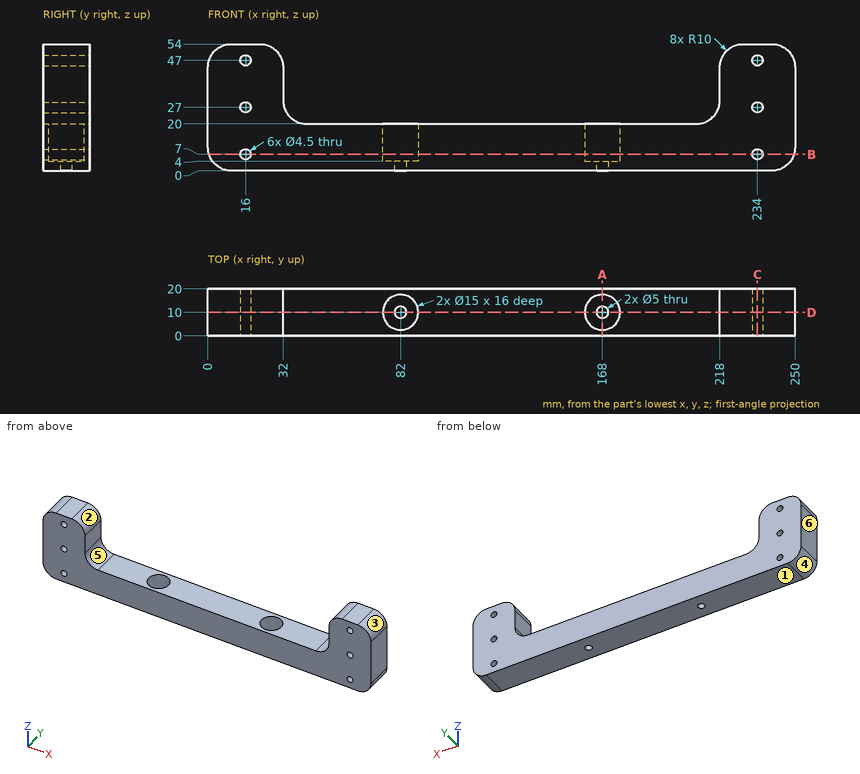
Can you work these out from the drawing? Everything is in mm from the part's minimum corner. A direction names the side the tool comes from. Give positions to 0.01 mm unless a question says otherwise; leave off trailing zeros. Order: outer loops, then holes, each group sorted by start corner. A loop starts at its lowest first (then second) coordinate and runs counter-clockwise, first axis right, second up. Notation, with made-up numbers: M -37,51 L -23,51 A30 cw -23,90 Z; hole C 65.25,-5.75 d7. An arc over 180 degrees is marked long. Use a Markdown table: item, result. Add a question column.
1. For pin 1 Ø5 at (y, z) = (17, 5.5) entering from +X; pin 2 Ø7.5 at (x, y) = (166.5, 9.5) entering from +Z, each with a flat end and sliding along its axis, tell me the tip position at first contact or that it passes through.
2. I need wall thicknesses on probe 1 along Z at (x, y) = (234, 15.25); probe 2 along X at (y, z) = (5.25, 33); probe 3 along Y at (x, z) = (168, 12). Which ranges of each line are inside material? Lowest first, please. Write a range as from..to.
3. Suppose I cut it at D-D (y = 10). Give the number of separate pieces and of enclosed holes in the cut face, and give its area (3 significant figures).
4. Suppose I cut it at A-A (x = 168). List the corners of the cut face in (y, z) for me, and give its area (3 significant figures).
5. Suppose I cut it at B-B (z = 7). List the corners of the cut face in (x, y) for me, and give its area (3 significant figures).
6. If we mould it in two halves opening along X, with no side actions, what happens to the marked faces 1, 2, 3 and 4? For each: +X half, -X half, draft (parallel to the pull), parting line (faces both ways), or undercut.
7. Suppose I cut it at C-C (x = 234). List the corners of the cut face in (y, z) for me, and give its area (3 significant figures).
8. On a 3-axis mill with a long thin cutter (end or side, diameter ignored), from which of +Z, -Z, +X, -X, +Y, -Y can I reach the whole of each face in a straight line? I mean the marked faces 5 and 6. Say none if no direction works.
Results list:
| question | item | result |
|---|---|---|
| 1 | pin 1 | stops at x = 249.8 |
| 1 | pin 2 | stops at z = 4 |
| 2 | probe 1 | z = 0..4.75, 9.25..24.75, 29.25..44.75, 49.25..54 |
| 2 | probe 2 | x = 0..32, 218..250 |
| 2 | probe 3 | y = 0..2.5, 17.5..20 |
| 3 | separate pieces | 3 |
| 3 | enclosed holes | 6 |
| 3 | area | 6,470 mm² |
| 4 | outline | M 0,0 L 7.5,0 L 7.5,4 L 2.5,4 L 2.5,20 L 0,20 Z; M 12.5,0 L 20,0 L 20,20 L 17.5,20 L 17.5,4 L 12.5,4 Z |
| 4 | area | 140 mm² |
| 5 | outline | M 0.46,0 L 13.75,0 L 13.75,20 L 0.46,20 Z; M 18.25,0 L 231.75,0 L 231.75,20 L 18.25,20 Z; M 236.25,0 L 249.54,0 L 249.54,20 L 236.25,20 Z; hole C 82,10 d15; hole C 168,10 d15 |
| 5 | area | 4,450 mm² |
| 6 | face 1 | draft |
| 6 | face 2 | undercut |
| 6 | face 3 | +X half |
| 6 | face 4 | -X half |
| 7 | outline | M 0,0 L 20,0 L 20,4.75 L 0,4.75 Z; M 0,9.25 L 20,9.25 L 20,24.75 L 0,24.75 Z; M 0,29.25 L 20,29.25 L 20,44.75 L 0,44.75 Z; M 0,49.25 L 20,49.25 L 20,54 L 0,54 Z |
| 7 | area | 810 mm² |
| 8 | face 5 | +Z, +Y, -Y |
| 8 | face 6 | +Z, -Z, -X, +Y, -Y |
